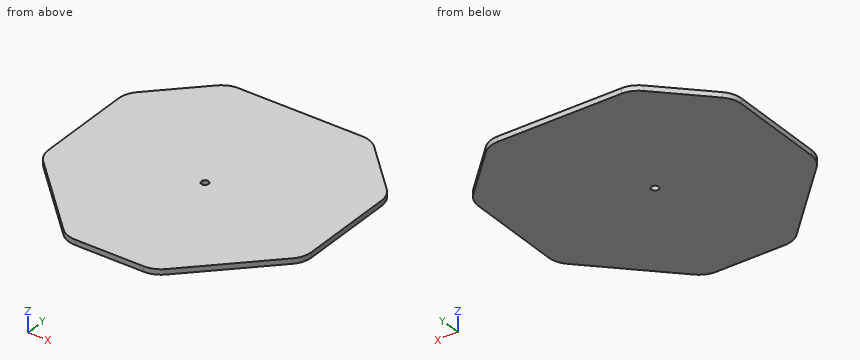
```python
from build123d import *

# Parameters (mm, degrees)
BOSS_EXTRUDE1_DEPTH = 5.588
CAVITY1_OUTLINE_R   = 3.834765
CAVITY1_DEPTH       = 5.588


# Read off the part's stored shape, not the designer's step: Cavity1
with BuildPart() as part:
    # Sketch1 → Boss-Extrude1 (new body)
    with BuildSketch(Plane.XY):
        with BuildLine():
            Line((65.678975516, 61.334336478), (-65.678975516, 61.334336478))
            ThreePointArc((-65.678975516, 61.334336478), (-75.399134698, 59.400876604), (-83.639487758, 53.89484872))
            Line((-83.639487758, 53.89484872), (-132.260512242, 5.273824236))
            ThreePointArc((-132.260512242, 5.273824236), (-137.766540126, -2.966528824), (-139.7, -12.686688006))
            Line((-139.7, -12.686688006), (-139.7, -114.753454114))
            ThreePointArc((-139.7, -114.753454114), (-137.766540126, -124.473613296), (-132.260512242, -132.713966356))
            Line((-132.260512242, -132.713966356), (-54.348302834, -210.626175764))
            ThreePointArc((-54.348302834, -210.626175764), (-46.107949774, -216.132203648), (-36.387790592, -218.065663522))
            Line((-36.387790592, -218.065663522), (36.387790592, -218.065663522))
            ThreePointArc((36.387790592, -218.065663522), (46.107949774, -216.132203648), (54.348302834, -210.626175764))
            Line((54.348302834, -210.626175764), (132.260512242, -132.713966356))
            ThreePointArc((132.260512242, -132.713966356), (137.766540126, -124.473613296), (139.7, -114.753454114))
            Line((139.7, -114.753454114), (139.7, -12.686688006))
            ThreePointArc((139.7, -12.686688006), (137.766540126, -2.966528824), (132.260512242, 5.273824236))
            Line((132.260512242, 5.273824236), (83.639487758, 53.89484872))
            ThreePointArc((83.639487758, 53.89484872), (75.399134698, 59.400876604), (65.678975516, 61.334336478))
        make_face()
    extrude(amount=BOSS_EXTRUDE1_DEPTH)

    # Cavity1 outline → Cavity1 (cut)
    with BuildSketch(Plane.XY):
        with Locations((0, -78.365663522)):
            Circle(CAVITY1_OUTLINE_R)
    extrude(amount=CAVITY1_DEPTH, mode=Mode.SUBTRACT)


solid = part.part
```
Geometry check sheet. Reference: the model listing, model coordinates, mm. Give positions to 0.01 mm unless a question says otherwise; leave off trailing zeros. Order: outer loops, then holes, each group sorted by start corner. A loop starts at its lowest first (then second) coordinate and runs counter-clockwise, first axis right, second up.
1. Thickness scan on L1, parallel to Y at x = 0, z = 3.6; L2, parallel to Y at x = 1.5, z = 5; L3, parallel to Y at x = -36.5, z = 2.45. Record the ranges inside material, lowest first.
2. Section check B-B, the plane z = 4.4. Enter the section's corners in (x, y), and give its area (3 significant figures).
3. Section check C-C, the plane y = 44. Enter the section's corners in (x, z).
4. Section check D-D, the plane x = -69. Enter the section's corners in (y, z), and give its area (3 significant figures).
5. Gauge pin test, flat ends, axial feed: pin 1 Ø3 at (x, z) = (93.5, 4) entering from -Y; pin 2 Ø3 at (x, z) = (-110.5, 4) entering from -Y; pin 3 Ø1.5 at (x, z) = (96, 1.5) entering from -Y. Record the tip position at first contact, or that the pin passes through.
6. Section check A-A, the plane x = 0. Enter the section's corners in (y, z).
Values follow:
1. L1: y = -218.07 to -82.2, -74.53 to 61.33
1. L2: y = -218.07 to -81.89, -74.84 to 61.33
1. L3: y = -218.07 to 61.33
2. outline: (-139.7, -114.75) arc R25.4 ccw to (-132.26, -132.71) - (-54.35, -210.63) arc R25.4 ccw to (-36.39, -218.07) - (36.39, -218.07) arc R25.4 ccw to (54.35, -210.63) - (132.26, -132.71) arc R25.4 ccw to (139.7, -114.75) - (139.7, -12.69) arc R25.4 ccw to (132.26, 5.27) - (83.64, 53.89) arc R25.4 ccw to (65.68, 61.33) - (-65.68, 61.33) arc R25.4 ccw to (-83.64, 53.89) - (-132.26, 5.27) arc R25.4 ccw to (-139.7, -12.69) - close; hole circle Ø7.67 at (0, -78.37)
2. area: 65,300 mm2
3. outline: (-93.53, 0) - (93.53, 0) - (93.53, 5.59) - (-93.53, 5.59) - close
4. outline: (-195.97, 0) - (61.12, 0) - (61.12, 5.59) - (-195.97, 5.59) - close
4. area: 1,440 mm2
5. pin 1: stops at y = -172.97
5. pin 2: stops at y = -155.97
5. pin 3: stops at y = -169.72
6. outline: (-218.07, 0) - (-82.2, 0) - (-82.2, 5.59) - (-218.07, 5.59) - close; (-74.53, 0) - (61.33, 0) - (61.33, 5.59) - (-74.53, 5.59) - close
